Answer from the drawing. Dimensions are ordinates in mm from the lowest x, y and z of the part. Round coordinates to 2 decimals unless told otherwise and drop trailing zeros. Order: outer loops, then holes, each group sorted by start corner. A loop starts at its lowest first (then second) coordinate and runs counter-clockwise, first axis right, second up. Notation, with made-up numbers: (33, 69.5) -> (87, 69.5) arc R22 cw to (87, 95.5) -> close; hole circle Ø2 at (-3.75, -34). An arc over 180 degrees is marked (long way). Use a Markdown table: item, result. Add a question column.
1. Consider L1, parallel to Y at x = 32.5, z = 1.6 (1 decimal); L2, parallel to X at y = 6.5, z = 2.1 (1 decimal); L3, parallel to Z at x = 63, y = 34.5. Determine where each line is inside the solid, lowest interval first. Write a range as [from, to].
2. Section D-D, the plane y = 20 is taken. Give the vertices of the cut face in (x, z).
3. The mould has two halves that part along Y. Classify the marked faces 1 and 2: +Y half, -Y half, draft (parallel to the pull), parting line (faces both ways), or undercut.
4. Given pin 1 (12 mm diameter, centred on x = 8.5, y = 5.5, fed in from +Z); pin 2 (23.5 mm diameter, centred on x = 36, y = 26.5, fed in from +Z), each flat-ended and moving along its own axis, determine where each tip first touches the part or whether it passes through.
5. Section C-C, the plane y = 36.5 is taken. Give the vertices of the cut face in (x, z) (1 decimal).
6. Section B-B, the plane x = 21.5 is taken. Give the vertices of the cut face in (y, z) (1 decimal).
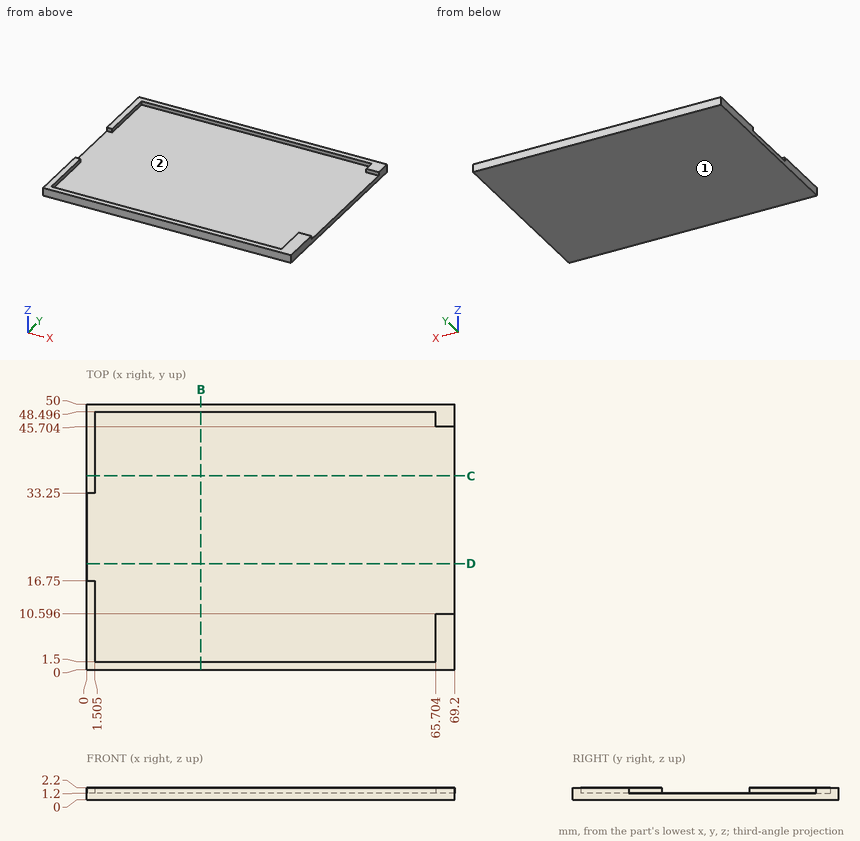
Verdict:
| question | item | result |
|---|---|---|
| 1 | L1 | y = [0, 1.5], [48.5, 50] |
| 1 | L2 | x = [0, 1.5], [65.7, 69.2] |
| 1 | L3 | z = [0, 1.2] |
| 2 | outline | (0, 0) -> (69.2, 0) -> (69.2, 1.2) -> (0, 1.2) -> close |
| 3 | face 1 | draft |
| 3 | face 2 | undercut |
| 4 | pin 1 | stops at z = 2.2 |
| 4 | pin 2 | stops at z = 1.2 |
| 5 | outline | (0, 0) -> (69.2, 0) -> (69.2, 1.2) -> (1.5, 1.2) -> (1.5, 2.2) -> (0, 2.2) -> close |
| 6 | outline | (0, 0) -> (50, 0) -> (50, 2.2) -> (48.5, 2.2) -> (48.5, 1.2) -> (1.5, 1.2) -> (1.5, 2.2) -> (0, 2.2) -> close |
